For this review, use the dimensioned drawing (mm, ordinates from the lowest corner) and the shaded views. A direction names the side the tool comes from. Round coordinates to 2 decimals unless told otherwise and drop trailing zeros. Loops run counter-clockwise (first coordinate to the right, second up) from the corner with the lowest first, then second, coordinate; pieces in that order, holes last. Notation, with made-up numbers: (63.25, -29.75) -> (95.25, -29.75) arc R21 cw to (95.25, -0.75) -> close; hole circle Ø5 at (27.25, -11.75). An arc over 180 degrees is marked (long way). Answer as CSV lines item,"result". Start each with the question number.
(1) Take a section at D-D, the plane x = 30. Write out the cut boundary in (y, z).
(2) Take a section at B-B, the plane z = 33. Write out the cut boundary in (x, y), and give its area (3 significant figures).
(3) For P1, Ø11, axis at x = 30, y = 140, coming from the +Z side, flat-tipped, find the tip position at first contact; note if it passes through.
(4) Draft analysis for pull direction X (two halves, no side actions). For the marked faces 3, 4 and 5, state which applies: +X half, -X half, draft (parallel to the pull), parting line (faces both ways), or undercut.
(5) Take a section at C-C, the plane x = 52. Write out the cut boundary in (y, z).
(6) To check wall thickness, follow line 1 (X direction, y = 160, z = 4.5); line 2 (Y direction, x = 30, z = 57.9). State the ranges of each line that lie inside material, in increasing order. Write a range as from..to.
(7) Take a section at A-A, the plane y = 90.5. Write out the cut boundary in (x, z).
(8) Machinability: for the marked faces 1 and 2, which of the approach directions +Z, -Z, +X, -X, +Y, -Y give a long, thin tool a straight path to every point of the face, cutting with its end or side? Answer none if there is none.
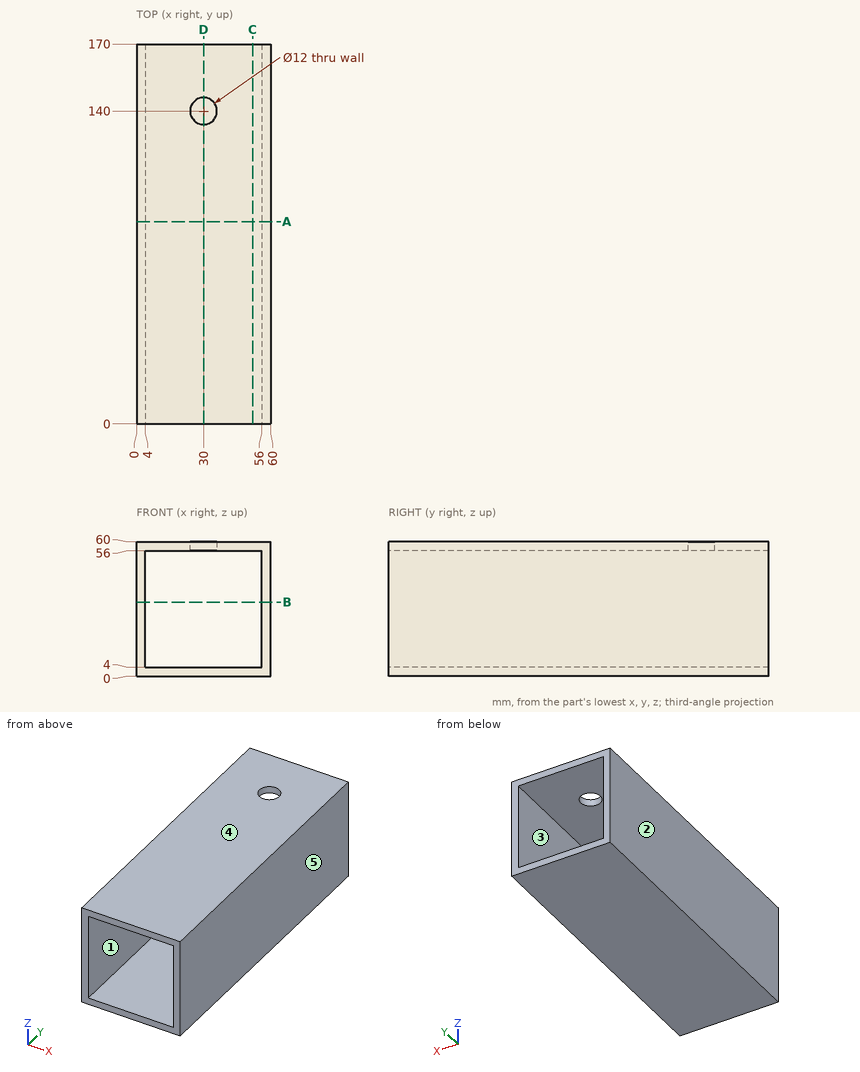
The answers:
1,outline,"(0, 0) -> (170, 0) -> (170, 4) -> (0, 4) -> close; (0, 56) -> (134, 56) -> (134, 60) -> (0, 60) -> close; (146, 56) -> (170, 56) -> (170, 60) -> (146, 60) -> close"
2,outline,"(0, 0) -> (4, 0) -> (4, 170) -> (0, 170) -> close; (56, 0) -> (60, 0) -> (60, 170) -> (56, 170) -> close"
2,area,"1,360 mm²"
3,P1,"z = 4"
4,face 3,"undercut"
4,face 4,"draft"
4,face 5,"+X half"
5,outline,"(0, 0) -> (170, 0) -> (170, 4) -> (0, 4) -> close; (0, 56) -> (170, 56) -> (170, 60) -> (0, 60) -> close"
6,line 1,"0..4, 56..60"
6,line 2,"0..134, 146..170"
7,outline,"(0, 0) -> (60, 0) -> (60, 60) -> (0, 60) -> close; hole (4, 4) -> (56, 4) -> (56, 56) -> (4, 56) -> close"
8,face 1,"+Y, -Y"
8,face 2,"+Z, -Z, -X, +Y, -Y"
